Verification items for the finished model (mm, model axes). A direction names the side the tool comes from. Coordinates: 2 decimals unless noted, no trailing zeros. Write each loop counter-clockwise with the first axis right and the second up, starting at its lowest first coordinate (ties: lowest second). Pieces come first, ordered by that corner, then holes. Notation, with made-up numbers: M -23,54.5 L 12,54.5 A12 ccw 12,77.5 Z; hole C 80.25,-15.5 d7. An arc over 180 degrees is marked long. One line per item, written item: value.
```python
from build123d import *

# Parameters (mm, degrees)
F1_DEPTH = 100
F2_R     = 1


# Not quite as in the source:
# - a feature names something its author has since deleted; it is built from what else it names


with BuildPart() as f1:
    # F0 (on Top) → F1 (new body)
    with BuildSketch(Plane.XY):
        with BuildLine():
            Line((-25, 50), (-25, -50))
            Line((-25, -50), (25, -50))
            Line((25, -50), (25, -45))
            Line((25, -45), (-12.5, -45))
            ThreePointArc((-12.5, -45), (-17.8033008589, -42.8033008589), (-20, -37.5))
            Line((-20, -37.5), (-20, 50))
            Line((-20, 50), (-25, 50))
        make_face()
    extrude(amount=F1_DEPTH)

    # F2
    f2_edges = [f1.edges().sort_by_distance(p)[0] for p in [
        (-20, 50, 50),
        (25, -45, 50),
    ]]
    fillet(f2_edges, radius=F2_R)


solid = f1.part
```
Item 1: Access from +Z, -Z, +X, -X, +Y, -Y to the whole of each face (thin tool, end or side, straight path). Record for faces 1 (the face through (6, -45, 49)), 2 (the face through (-20.5, -10.9, 100)).
The answers:
face 1: +Z, -Z, +X, +Y
face 2: +Z, +X, -X, +Y, -Y
Item 2: Cross-section at B-B, the plane y = -42. Enter the section's corners in (x, z), and give its area (3 significant figures).
The answers:
outline: M -25,0 L -18.5,0 L -18.5,100 L -25,100 Z
area: 650 mm²
Item 3: Cross-section at C-C, the plane x = 16.5. Enter the section's corners in (y, z), and give its area (3 significant figures).
The answers:
outline: M -50,0 L -45,0 L -45,100 L -50,100 Z
area: 500 mm²
Item 4: Cross-section at A-A, the plane z = 89. Enter the section's corners in (x, y).
The answers:
outline: M -25,-50 L 25,-50 L 25,-46 A1 ccw 24,-45 L -12.5,-45 A7.5 cw -20,-37.5 L -20,49 A1 ccw -21,50 L -25,50 Z
Item 5: Scan lines: line 1 (Y direction, x = -13, z = 49); line 2 (X direction, y = -6, z = 88.5); line 3 (Y direction, x = -19, z = 91). Record each from-to range of solid material in increasing order.
The answers:
line 1: y = -50 to -44.98
line 2: x = -25 to -20
line 3: y = -50 to -41.24
Item 6: Go/stop test with flat-tipped pins: P1, Ø6, axis at y = -38.5, z = 24, coming from the +X side; P2, Ø12, axis at y = -30.5, z = 53.5, coming from the +X side. Record where each tip stops, or that it passes through.
The answers:
P1: stops at x = -18.84
P2: stops at x = -20
